from build123d import *

# Parameters (mm, degrees)
ESQUISSE1_W             = 60
ESQUISSE1_H             = 60
BOSS_EXTRU_1_DEPTH      = 60
ESQUISSE2_R             = 6
ENL_V_MAT_EXTRU_1_DEPTH = 20
ESQUISSE3_R             = 6
ENL_V_MAT_EXTRU_2_DEPTH = 20


with BuildPart() as part:
    # Esquisse1 → Boss.-Extru.1 (new body)
    with BuildSketch(Plane(origin=(0, 0, 0), x_dir=(1, 0, 0), z_dir=(0, 1, 0))):
        with Locations((30, 30)):
            Rectangle(ESQUISSE1_W, ESQUISSE1_H)
    extrude(amount=BOSS_EXTRU_1_DEPTH)

    # Esquisse2 → Enlèv. mat.-Extru.1 (cut)
    with BuildSketch(Plane.XY):
        with Locations((30, 30)):
            Circle(ESQUISSE2_R)
    extrude(amount=-ENL_V_MAT_EXTRU_1_DEPTH, mode=Mode.SUBTRACT)

    # Esquisse3 → Enlèv. mat.-Extru.2 (cut)
    with BuildSketch(Plane.ZY):
        with Locations((-30, 30)):
            Circle(ESQUISSE3_R)
    extrude(amount=-ENL_V_MAT_EXTRU_2_DEPTH, mode=Mode.SUBTRACT)


solid = part.part
Can you work these out from the model? Positions are in its coordinate system, mm. A direction names the side the tool comes from. Coordinates: 2 decimals unless noted, no trailing zeros. Order: outer loops, then holes, each group sorted by start corner. A loop starts at its lowest first (then second) coordinate and runs counter-clockwise, first axis right, second up. Notation, with made-up numbers: M 16,12 L 39,12 A32 cw 39,46 Z; hole C -8.75,-16 d3. An arc over 180 degrees is marked long. Write item = value, one per line.
(1) For faces 5 (the face through (20, 30, -30)), 6 (the face through (30, 30, -60)), 7 (the face through (30, 30, -20)), which set-ups out of +Z, -Z, +X, -X, +Y, -Y let a thin tool reach every point of the face, with its end or its side?
Results are:
face_5 = -X
face_6 = -Z, +X, -X, +Y, -Y
face_7 = +Z
(2) I need wall thicknesses on line 1 along X through (y, z) = (25.5, -18). Which ranges of the line are inside material? Lowest first, please. Write a range as [from, to].
Results are:
line_1 = [0, 26.03], [33.97, 60]
(3) Suppose I cut it at B-B on x = 18. Please give me the cut outline in (y, z).
Results are:
outline = M 0,-60 L 60,-60 L 60,0 L 0,0 Z; hole C 30,-30 d12
(4) Suppose I cut it at C-C on z = -31. Please give me the cut outline in (x, y), plus the area to 3 significant figures.
Results are:
outline = M 0,0 L 60,0 L 60,60 L 0,60 L 0,35.92 L 20,35.92 L 20,24.08 L 0,24.08 Z
area = 3,360 mm2
(5) Suppose I cut it at A-A on x = 30. Please give me the cut outline in (y, z), plus the area to 3 significant figures.
Results are:
outline = M 0,-60 L 60,-60 L 60,0 L 36,0 L 36,-20 L 24,-20 L 24,0 L 0,0 Z
area = 3,360 mm2
(6) If we mould it in two halves opening along Y, with no side actions, what happens to faces 1 (the face through (30, 0, -30)), 2 (the face through (25.24, 26.35, -9.86)), 3 (the face through (23, 30, 0)), 4 (the face through (30, 60, -30))? For each: pulls with the +Y half, pulls with the -Y half, needs draft (parallel to the pull), parting line crosses it, or undercut.
Results are:
face_1 = pulls with the -Y half
face_2 = undercut
face_3 = needs draft
face_4 = pulls with the +Y half
(7) Suppose I cut it at D-D on z = -18. Please give me the cut outline in (x, y).
Results are:
outline = M 0,0 L 60,0 L 60,60 L 0,60 Z; hole C 30,30 d12
